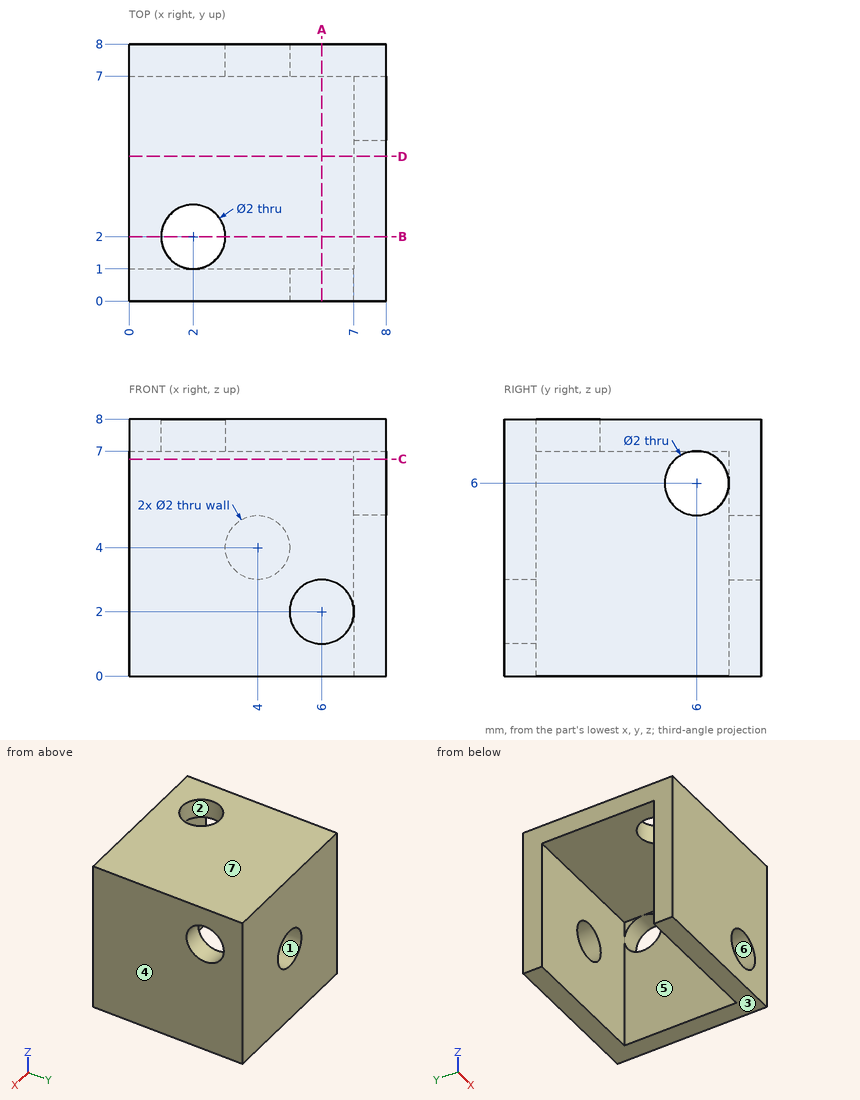
Geometry check sheet. Reference: drawing and pictorial views, mm from the part's lowest x, y, z. A direction names the side the tool comes from. Round coordinates to 2 decimals unless told otherwise and drop trailing zeros. Loops run counter-clockwise (first coordinate to the right, second up) from the corner with the lowest first, then second, coordinate; pieces in that order, holes last.
1. Sectioned sample at B-B on y = 2. Record the boundary of the cut face in (x, z), and give its area (3 significant figures).
2. Sectioned sample at A-A on x = 6. Record the boundary of the cut face in (y, z).
3. Set-up check for the marked faces 5, 6 and 7: record each of +Z, -Z, +X, -X, +Y, -Y from which the full face is reachable in a straight line by a thin tool's end or side.
4. Scan lines: probe 1 along Y at (x, z) = (1, 6); probe 2 along Y at (x, z) = (7.35, 6); probe 3 along Z at (x, y) = (4, 7.65). Record each from-to range of solid material in increasing order.
5. Mould release check, pull along X, two halves, no side actions. Record for the marked faces 1, 2, 3 and 4: released by +X, released by -X, zero draft, split by the parting line, or undercut.
6. Sectioned sample at C-C on z = 6.75. Record the boundary of the cut face in (x, y).
7. Sectioned sample at D-D on y = 4.5. Record the boundary of the cut face in (x, z), and give its area (3 significant figures).
Recorded:
1. outline: (0, 7) - (1, 7) - (1, 8) - (0, 8) - close; (3, 7) - (7, 7) - (7, 0) - (8, 0) - (8, 8) - (3, 8) - close
1. area: 13.0 mm2
2. outline: (0, 0) - (1, 0) - (1, 1) - (0, 1) - close; (0, 3) - (1, 3) - (1, 7) - (7, 7) - (7, 0) - (8, 0) - (8, 8) - (0, 8) - close
3. face 5: -Z, -X
3. face 6: -Y
3. face 7: +Z, +X, -X, +Y, -Y
4. probe 1: y = 0 to 1, 7 to 8
4. probe 2: y = 0 to 5, 7 to 8
4. probe 3: z = 0 to 3, 5 to 8
5. face 1: undercut
5. face 2: undercut
5. face 3: zero draft
5. face 4: released by +X
6. outline: (0, 0) - (8, 0) - (8, 5.34) - (7, 5.34) - (7, 1) - (0, 1) - close; (0, 7) - (7, 7) - (7, 6.66) - (8, 6.66) - (8, 8) - (0, 8) - close
7. outline: (0, 7) - (7, 7) - (7, 0) - (8, 0) - (8, 8) - (0, 8) - close
7. area: 15.0 mm2
